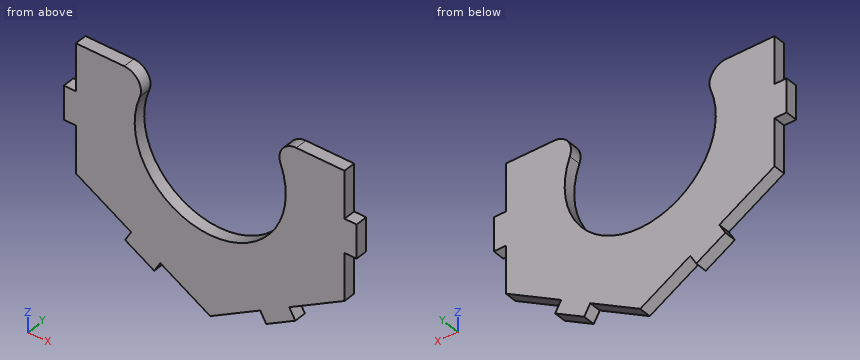
from build123d import *

# Parameters (mm, degrees)
BOSS_EXTRUDE1_DEPTH = 4.572
SKETCH2_W           = 4.572
SKETCH2_H           = 12.7
BOSS_EXTRUDE2_DEPTH = 4.572


with BuildPart() as part:
    # Sketch1 → Boss-Extrude1 (new body)
    with BuildSketch(Plane(origin=(0, 0, 0), x_dir=(1, 0, 0), z_dir=(0, 1, 0))):
        with BuildLine():
            Line((-50.8, -19.05), (-32.534068682, -19.05))
            ThreePointArc((-32.534068682, -19.05), (-27.290728751, -16.281883075), (-26.618783467, -10.390909091))
            ThreePointArc((-26.618783467, -10.390909091), (0, 28.575), (26.618783467, -10.390909091))
            ThreePointArc((26.618783467, -10.390909091), (27.290728751, -16.281883075), (32.534068682, -19.05))
            Line((32.534068682, -19.05), (50.8, -19.05))
            Line((50.8, -19.05), (50.8, 29.329393675))
            Line((50.8, 29.329393675), (0, 58.65878735))
            Line((0, 58.65878735), (-50.8, 29.329393675))
            Line((-50.8, 29.329393675), (-50.8, -19.05))
        make_face()
    extrude(amount=BOSS_EXTRUDE1_DEPTH)

    # Sketch2 → Boss-Extrude2 (add)
    with BuildSketch(Plane(origin=(0, 4.572, 0), x_dir=(1, 0, 0), z_dir=(0, 1, 0))):
        with Locations((-53.086, 5.139696837)):
            Rectangle(SKETCH2_W, SKETCH2_H)
        Polygon((-29.902807007, 41.394393675), (-32.188807007, 45.353861821), (-21.190284379, 51.703861821), (-18.904284379, 47.744393675), align=None)
        Polygon((18.904284379, 47.744393675), (21.190284379, 51.703861821), (32.188807007, 45.353861821), (29.902807007, 41.394393675), align=None)
        with Locations((53.086, 5.139696837)):
            Rectangle(SKETCH2_W, SKETCH2_H)
    extrude(amount=-BOSS_EXTRUDE2_DEPTH)


solid = part.part
Could you check a few things on this model? Use its own coordinates, in mm. Give positions to 0.01 mm unless a question says otherwise; leave off trailing zeros. Order: outer loops, then holes, each group sorted by start corner. A loop starts at its lowest first (then second) coordinate and runs counter-clockwise, first axis right, second up. Notation, with made-up numbers: (25.25, 39) - (58.25, 39) arc R23 ccw to (58.25, 51) - close; hole circle Ø2 at (28.5, 59). An arc over 180 degrees is marked (long way). One line per question, with ' | ' between items. Start each with the question number.
Item 1: I want a section at D-D on x = -8. Write out the boundary of the cut face in (y, z), then the cut area to 3 significant figures.
Item 2: I need wall thicknesses on probe 1 along X at (y, z) = (1.4, 0) (3 decimals); probe 2 along X at (y, z) = (4.25, -15); probe 3 along X at (y, z) = (1.45, -40). Which ranges of each line are inside material? Lowest first, please. Write a range as [from, to].
Item 3: I'm going to push flat-ended pins straight in: pin 1 Ø2 at (x, y) = (15.5, 3) entering from -Z; pin 2 Ø2 at (y, z) = (3, -46) entering from -X; pin 3 Ø1.4 at (x, y) = (52.5, 3) entering from +Z. Where does each tip first touch, or does it pass through?
Item 4: I want a section at C-C on y = 2.25. Write out the boundary of the cut face in (x, z) (3 decimals).
Item 5: I want a section at B-B on z = -21. Write out the boundary of the cut face in (x, y).
Item 6: I want a section at A-A on z = 0. Write out the boundary of the cut face in (x, y) (3 decimals), then the cut area to 3 significant figures.
Verdict:
1) outline: (0, -54.04) - (4.57, -54.04) - (4.57, -27.43) - (0, -27.43) - close | area: 122 mm^2
2) probe 1: [-55.372, -28.575], [28.575, 55.372] | probe 2: [-50.8, -24.32], [24.32, 50.8] | probe 3: [-32.32, 32.32]
3) pin 1: z = -50.29 | pin 2: x = -32.19 | pin 3: z = 1.21
4) outline: (-55.372, -11.49) - (-50.8, -11.49) - (-50.8, -29.329) - (-29.903, -41.394) - (-32.189, -45.354) - (-21.19, -51.704) - (-18.904, -47.744) - (0, -58.659) - (18.904, -47.744) - (21.19, -51.704) - (32.189, -45.354) - (29.903, -41.394) - (50.8, -29.329) - (50.8, -11.49) - (55.372, -11.49) - (55.372, 1.21) - (50.8, 1.21) - (50.8, 19.05) - (32.534, 19.05) arc R6.35 ccw to (26.619, 10.391) arc R28.575 cw (long way) to (-26.619, 10.391) arc R6.35 ccw to (-32.534, 19.05) - (-50.8, 19.05) - (-50.8, 1.21) - (-55.372, 1.21) - close
5) outline: (-50.8, 0) - (-19.38, 0) - (-19.38, 4.57) - (-50.8, 4.57) - close; (19.38, 0) - (50.8, 0) - (50.8, 4.57) - (19.38, 4.57) - close
6) outline: (-55.372, 0) - (-28.575, 0) - (-28.575, 4.572) - (-55.372, 4.572) - close; (28.575, 0) - (55.372, 0) - (55.372, 4.572) - (28.575, 4.572) - close | area: 245 mm^2
